Here's how the part is built. I have some questions about the finished solid (model axes, mm). A direction names the side the tool comes from. Round coordinates to 2 decimals unless told otherwise and drop trailing zeros. Write each loop counter-clockwise with the first axis right and the second up, starting at its lowest first coordinate (ties: lowest second). Pieces come first, ordered by that corner, then holes. Notation, with made-up numbers: M -34,41.25 L -20,41.25 A22 ccw -20,77.25 Z; hole C -1.75,14.5 d11. An arc over 180 degrees is marked long. Write item = value, one per line. Start each with the question number.
(1) On a 3-axis mill with a long thin cutter (end or side, diameter ignored), from which of +Z, -Z, +X, -X, +Y, -Y can I reach the whole of each face in a straight line? I mean faces 5 (the flat face through (0, 0, 3)), 6 (the cylindrical face through (-32.47, -1.43, 3.45)). Say none if no direction works.
(2) I want a section at B-B (x = 0). List the corners of the cut face in (y, z) for me, and give its area (3 significant figures).
(3) Will these pins go through, and if not, where does the flat tip stop? pin 1 Ø2 at (x, y) = (-4.5, 12.5) entering from -Z; pin 2 Ø13.5 at (x, y) = (0, 0) entering from +Z; pin 3 Ø4 at (x, z) = (22, 5.5) entering from +Y; pin 4 Ø3 at (x, z) = (27, 3.5) entering from +Y.
(4) I want a section at A-A (y = 0). List the corners of the cut face in (x, z) for me.
(5) If we mould it in two halves opening along Y, with no side actions, what happens to faces 1 (the cylindrical face through (-5.99, -45.61, 4.72)), 2 (the cylindrical face through (41.53, -1.43, 3.45)), 3 (the cylindrical face through (-7.493, 0.33, 5.028)), 4 (the flat face through (-1, 1, 0))? For each: released by +Y, released by -Y, zero draft, split by the parting line, or undercut.
(6) I need wall thicknesses on line 1 along Y through (x, z) = (0, 5.05); line 2 along Y through (x, z) = (-6, 4.25); line 3 along Y through (x, z) = (-15, 5). Which ranges of each line are inside material? Lowest first, please.
Autodesk Inventor part; units mm, degrees
ref_plane "YZ Plane" through (0, 0, 0) normal (1, 0, 0) x (0, 1, 0)
ref_plane "XZ Plane" through (0, 0, 0) normal (0, 1, 0) x (-1, 0, 0)
ref_plane "XY Plane" through (0, 0, 0) normal (0, 0, 1) x (1, 0, 0)
sketch "Sketch1" plane through (0, 0, 0) normal (0, 0, 1) x (1, 0, 0)
  circle A0 centre (0, 0) radius 46
  circle A1 centre (-37, 0) radius 4.75
  circle A2 centre (37, 0) radius 4.75
  dimension "d0" = 92
  dimension "d7" = 9.5
  dimension "d8" = 9.5
  dimension "d9" = 74
  dimension "d10" = 37
extrude "Extrusion1" add sketch "Sketch1" along normal blind 7
sketch "Sketch2" plane through (0, 0, 7) normal (0, 0, 1) x (1, 0, 0)
  circle A0 centre (0, 0) radius 46
  circle A1 centre (0, 0) radius 7.5
  dimension "d3" = 15
extrude "Extrusion2" cut sketch "Sketch2" against normal blind 4 contours A1
fillet "Fillet1" radius 2.5 1 edges at (-46, 0, 0)
properties part number "ANTI-SKID PAD 100mm WITH ATTACHMENT BORES" material "Rubber"
Returned:
q1.face_5 = +Z
q1.face_6 = +Z, -Z
q2.outline = M -46,2.5 A2.5 ccw -43.5,0 L 43.5,0 A2.5 ccw 46,2.5 L 46,7 L 7.5,7 L 7.5,3 L -7.5,3 L -7.5,7 L -46,7 Z
q2.area = 581 mm²
q3.pin_1 = 0
q3.pin_2 = 3
q3.pin_3 = 41.42
q3.pin_4 = 38.29
q4.outline = M -46,2.5 A2.5 ccw -43.5,0 L -41.75,0 L -41.75,7 L -46,7 Z; M -32.25,0 L 32.25,0 L 32.25,7 L 7.5,7 L 7.5,3 L -7.5,3 L -7.5,7 L -32.25,7 Z; M 41.75,0 L 43.5,0 A2.5 ccw 46,2.5 L 46,7 L 41.75,7 Z
q5.face_1 = split by the parting line
q5.face_2 = undercut
q5.face_3 = undercut
q5.face_4 = zero draft
q6.line_1 = -46 to -7.5, 7.5 to 46
q6.line_2 = -45.61 to -4.5, 4.5 to 45.61
q6.line_3 = -43.49 to 43.49
